from build123d import *

# Parameters (mm, degrees)
RESSALTO_EXTRUS_O1_DEPTH = 40
ESBO_O2_W                = 60
ESBO_O2_H                = 60
RESSALTO_EXTRUS_O2_DEPTH = 20


with BuildPart() as part:
    # Esboço1 → Ressalto-extrusão1 (new body)
    with BuildSketch(Plane.XY):
        Polygon((0, 0), (60, 0), (60, 20), (20, 60), (0, 60), align=None)
    extrude(amount=RESSALTO_EXTRUS_O1_DEPTH)

    # Esboço2 → Ressalto-extrusão2 (add)
    with BuildSketch(Plane(origin=(0, 0, 0), x_dir=(-1, 0, 0), z_dir=(0, 0, -1))):
        with Locations((-30, 30)):
            Rectangle(ESBO_O2_W, ESBO_O2_H)
    extrude(amount=RESSALTO_EXTRUS_O2_DEPTH)


solid = part.part
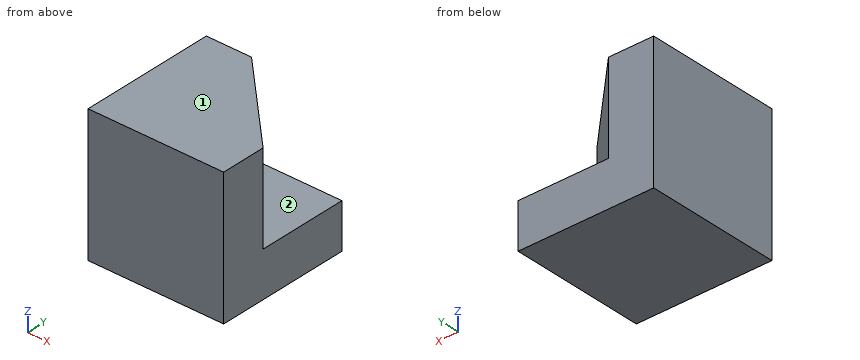
Geometry: final body of the model. Coordinates: model frame, mm. Face numbers are marked on the shaded views. A direction names the side the tool comes from. Round coordinates to 2 decimals unless told otherwise and drop trailing zeros. Order: outer loops, then holes, each group sorted by start corner. A loop starts at its lowest first (then second) coordinate and runs counter-clockwise, first axis right, second up. Notation, with made-up numbers: (31, 7.25) -> (58, 7.25) arc R23 ccw to (58, 36.25) -> close; hole circle Ø2 at (-24.5, 32.5). An arc over 180 degrees is marked (long way). Put each result on its own line as item: value. Start each with the question number.
Q1. Section C-C on z = 9.5. Return the cut outline in (x, y), and give its area (3 significant figures).
Q2. First-contact query: pin 1 (2 mm diameter, centred on y = 31.5, z = 9.5, fed in from -X). Flat tip, straight axial feed; report the tip coordinate or a pass-through.
Q3. Section B-B on x = 36. Return the cut outline in (y, z).
Q4. Section A-A on y = 43.5. Return the cut outline in (x, z), and give its area (3 significant figures).
Q5. Line query: probe 1 along Z at (x, y) = (52, 55.5); probe 2 along X at (y, z) = (56.5, 27); probe 3 along X at (y, z) = (26, 23.5). Output: solid intervals per line, ascending.
Q6. Reachability of the marked faces 1 and 2 from +Z, -Z, +X, -X, +Y, -Y: full face, straight path, thin tool, end or side. Return the list, or none.
Ans:
1. outline: (0, 0) -> (60, 0) -> (60, 20) -> (20, 60) -> (0, 60) -> close
1. area: 2,800 mm2
2. pin 1: stops at x = 0
3. outline: (0, -20) -> (60, -20) -> (60, 0) -> (44, 0) -> (44, 40) -> (0, 40) -> close
4. outline: (0, -20) -> (60, -20) -> (60, 0) -> (36.5, 0) -> (36.5, 40) -> (0, 40) -> close
4. area: 2,660 mm2
5. probe 1: z = -20 to 0
5. probe 2: x = 0 to 23.5
5. probe 3: x = 0 to 54
6. face 1: +Z, +X, -X, +Y, -Y
6. face 2: +Z, +X, +Y
